Model file for the job. Use its own axes, mm. Face numbers are marked on the shaded views. A direction names the side the tool comes from. Round coordinates to 2 decimals unless told otherwise and drop trailing zeros. Loops run counter-clockwise (first coordinate to the right, second up) from the corner with the lowest first, then second, coordinate; pieces in that order, holes last. Notation, with made-up numbers: (-40, 3) - (15, 3) arc R38 cw to (15, 42) - close; hole circle Ø7 at (-16.5, 55). An arc over 180 degrees is marked (long way). Answer as a JSON object with one key per item and string values.
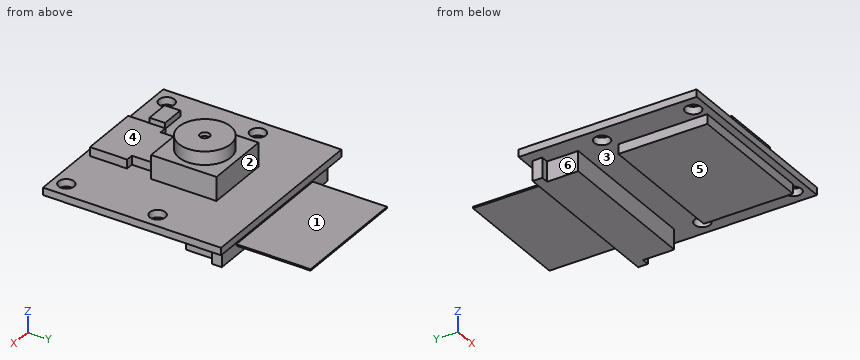
from build123d import *

# Parameters (mm, degrees)
SKICA1_W                 = 25.2
SKICA1_H                 = 24
SKICA1_R                 = 1.05
SKICA1_W_2               = 8.8
SKICA1_H_2               = 8.8
SKICA1_R_2               = 3.5
P_IDAT_VYSUNUT_M1_DEPTH  = 1
SKICA1_3_W               = 8.8
SKICA1_3_H               = 8.8
SKICA1_3_R               = 3.5
P_IDAT_VYSUNUT_M2_DEPTH  = 3.2
SKICA1_4_R               = 3.5
P_IDAT_VYSUNUT_M3_DEPTH  = 5
SKICA2_W                 = 8
SKICA2_H                 = 5
SKICA2_W_2               = 6
SKICA2_H_2               = 3.5
P_IDAT_VYSUNUT_M4_DEPTH  = 1.2
SKICA3_W                 = 20.1
SKICA3_H                 = 4.2
P_IDAT_VYSUNUT_M5_DEPTH  = 2.7
SKICA4_W                 = 17.9
SKICA4_H                 = 12
P_IDAT_VYSUNUT_M6_DEPTH  = 1.3
SKICA5_W                 = 3.2
SKICA5_H                 = 2.1
P_IDAT_VYSUNUT_M7_DEPTH  = 0.8
SKICA6_R                 = 0.65
ODEBRAT_VYSUNUT_M1_DEPTH = 0.5
SKICA7_W                 = 16
SKICA7_H                 = 0.2
P_IDAT_VYSUNUT_M9_DEPTH  = 10


with BuildPart() as part:
    # Skica1 → P_idat vysunut_m1 (new body)
    with BuildSketch(Plane.XY):
        Rectangle(SKICA1_W, SKICA1_H)
        with Locations((10.5, 2.1)):
            Circle(SKICA1_R, mode=Mode.SUBTRACT)
        with Locations((-10.5, 2.1)):
            Circle(SKICA1_R, mode=Mode.SUBTRACT)
        with Locations((10.5, -10.2)):
            Circle(SKICA1_R, mode=Mode.SUBTRACT)
        with Locations((-10.5, -10.2)):
            Circle(SKICA1_R, mode=Mode.SUBTRACT)
        with Locations((0, 1.7)):
            Rectangle(SKICA1_W_2, SKICA1_H_2, mode=Mode.SUBTRACT)
        with Locations((0, 1.7)):
            Rectangle(SKICA1_W_2, SKICA1_H_2)
        with Locations((0, 1.7)):
            Circle(SKICA1_R_2, mode=Mode.SUBTRACT)
        with Locations((0, 1.7)):
            Circle(SKICA1_R_2)
    extrude(amount=-P_IDAT_VYSUNUT_M1_DEPTH)

    # Skica1_3 → P_idat vysunut_m2 (add)
    with BuildSketch(Plane.XY):
        with Locations((0, 1.7)):
            Rectangle(SKICA1_3_W, SKICA1_3_H)
        with Locations((0, 1.7)):
            Circle(SKICA1_3_R, mode=Mode.SUBTRACT)
    extrude(amount=P_IDAT_VYSUNUT_M2_DEPTH)

    # Skica1_4 → P_idat vysunut_m3 (add)
    with BuildSketch(Plane.XY):
        with Locations((0, 1.7)):
            Circle(SKICA1_4_R)
    extrude(amount=P_IDAT_VYSUNUT_M3_DEPTH)

    # Skica2 → P_idat vysunut_m4 (add)
    with BuildSketch(Plane.XY):
        with Locations((0, -8.7)):
            Rectangle(SKICA2_W, SKICA2_H)
        with Locations((0, -4.45)):
            Rectangle(SKICA2_W_2, SKICA2_H_2)
    extrude(amount=P_IDAT_VYSUNUT_M4_DEPTH)

    # Skica3 → P_idat vysunut_m5 (add)
    with BuildSketch(Plane(origin=(0, 0, -1), x_dir=(-1, 0, 0), z_dir=(0, 0, -1))):
        with Locations((0, 7.7)):
            Rectangle(SKICA3_W, SKICA3_H)
        Polygon((-11.05, 9.8), (-10.05, 9.8), (10.05, 9.8), (11.05, 9.8), (11.05, 11.1), (-11.05, 11.1), align=None)
    extrude(amount=P_IDAT_VYSUNUT_M5_DEPTH)

    # Skica4 → P_idat vysunut_m6 (add)
    with BuildSketch(Plane(origin=(0, 0, -1), x_dir=(-1, 0, 0), z_dir=(0, 0, -1))):
        with Locations((-0.15, -5)):
            Rectangle(SKICA4_W, SKICA4_H)
    extrude(amount=P_IDAT_VYSUNUT_M6_DEPTH)

    # Skica5 → P_idat vysunut_m7 (add)
    with BuildSketch(Plane.XY):
        with Locations((-7.1, -8.25)):
            Rectangle(SKICA5_W, SKICA5_H)
    extrude(amount=P_IDAT_VYSUNUT_M7_DEPTH)

    # Skica6 → Odebrat vysunut_m1 (cut)
    with BuildSketch(Plane.XY.offset(5)):
        with Locations((0, 1.7)):
            Circle(SKICA6_R)
    extrude(amount=-ODEBRAT_VYSUNUT_M1_DEPTH, mode=Mode.SUBTRACT)

    # Skica7 → P_idat vysunut_m9 (add)
    with BuildSketch(Plane(origin=(0, 11.1, 0), x_dir=(1, 0, 0), z_dir=(0, 1, 0))):
        with Locations((0, 2.3)):
            Rectangle(SKICA7_W, SKICA7_H)
    extrude(amount=P_IDAT_VYSUNUT_M9_DEPTH)


solid = part.part
1) Probe probe 1 along Y at (x, z) = (-10.5, -0.25); probe 2 along Y at (x, z) = (-7.25, -2); probe 3 along Y at (x, z) = (0, 4.7). List the from-to ranges inside material, lowest first.
Values follow:
{"probe 1": "-12 to -11.25, -9.15 to 1.05, 3.15 to 12", "probe 2": "-11 to 1, 5.6 to 11.1", "probe 3": "-1.8 to 1.05, 2.35 to 5.2"}
2) Slice it at D-D on y = 8.5. List the corners of the cut face in (x, z), then the cut area to 3 significant figures.
Values follow:
{"outline": "(-12.6, -1) - (-10.05, -1) - (-10.05, -3.7) - (10.05, -3.7) - (10.05, -1) - (12.6, -1) - (12.6, 0) - (-12.6, 0) - close", "area": "79.5 mm²"}
3) Slice it at A-A on x = 10.5. List the corners of the cut face in (y, z).
Values follow:
{"outline": "(-12, -1) - (-11.25, -1) - (-11.25, 0) - (-12, 0) - close; (-9.15, -1) - (1.05, -1) - (1.05, 0) - (-9.15, 0) - close; (3.15, -1) - (9.8, -1) - (9.8, -3.7) - (11.1, -3.7) - (11.1, -1) - (12, -1) - (12, 0) - (3.15, 0) - close"}
4) Slice it at B-B on y = -10.2. List the corners of the cut face in (x, z).
Values follow:
{"outline": "(-12.6, -1) - (-11.55, -1) - (-11.55, 0) - (-12.6, 0) - close; (-9.45, -1) - (-8.8, -1) - (-8.8, -2.3) - (9.1, -2.3) - (9.1, -1) - (9.45, -1) - (9.45, 0) - (4, 0) - (4, 1.2) - (-4, 1.2) - (-4, 0) - (-9.45, 0) - close; (11.55, -1) - (12.6, -1) - (12.6, 0) - (11.55, 0) - close"}
5) Tool access for the marked faces 4, 5 and 6: list every direction of +Z, -Z, +X, -X, +Y, -Y with a clear straight run to the whole face (end or side of a thin tool).
Values follow:
{"face 4": "+Z, +X, -X, -Y", "face 5": "-Z, +X, -X, -Y", "face 6": "-Z, -X, -Y"}
6) Drop flat-ended pins along their axis: P1, Ø1, axis at y = -6.5, z = -2, coming from the -X side; P2, Ø1.5, axis at x = 9, y = -6, coming from the -Z side; P3, Ø0.5, axis at x = 6, z = -0.5, coming from the +Y side. Give the stop position or say it passes through.
Values follow:
{"P1": "x = -8.8", "P2": "z = -2.3", "P3": "y = 12"}
7) Two-plate mould, pull along Y, no slides. Class the marked faces 1, 2 and 3: pulls with the +Y half, pulls with the -Y half, needs draft (parallel to the pull), parting line crosses it, or undercut.
Values follow:
{"face 1": "needs draft", "face 2": "pulls with the +Y half", "face 3": "undercut"}
